The model under review builds one solid part; all positions refer to its coordinate system, in mm. A direction names the side the tool comes from. Give positions to 0.01 mm unless a question says otherwise; leave off trailing zeros. Order: outer loops, then holes, each group sorted by start corner. A loop starts at its lowest first (then second) coordinate and runs counter-clockwise, first axis right, second up. Notation, with made-up numbers: (19.25, -20) - (32.25, -20) arc R21 cw to (32.25, 14) - close; hole circle Ø5 at (-34.5, 64.5). An arc over 180 degrees is marked (long way). Put each result on its own line as item: value.
```python
from build123d import *

# Parameters (mm, degrees)
M4_TAPPED_HOLE1_D     = 3.3
M4_TAPPED_HOLE1_DEPTH = 6
M4_TAPPED_HOLE1_TIP   = 0.991420021
SKETCH6_W             = 40
SKETCH6_H             = 40
BOSS_EXTRUDE1_DEPTH   = 28.5
CUT_EXTRUDE1_REACH    = 124.315
CIRPATTERN1_COUNT     = 4
CHAMFER1_SIZE         = 0.4
BOSS_EXTRUDE2_DEPTH   = 1.5


with BuildPart() as part:
    # Sketch1 → Revolve1 (revolve)
    with BuildSketch(Plane.XY, mode=Mode.PRIVATE) as revolve1_sk:
        Polygon((0, 0), (0, 20), (64.5, 20), (64.5, 13), (66.5, 13), (66.5, 6), (67.5, 6), (67.5, 5), (90.5, 5), (90.5, 0), align=None)
    revolve(revolve1_sk.sketch.rotate(Axis((0, 0, 0), (1, 0, 0)), 90), axis=Axis((0, 0, 0), (1, 0, 0)))

    # M4 Tapped Hole1
    with Locations(Plane(origin=(64.5, 0, 0), x_dir=(0, 0, -1), z_dir=(1, 0, 0))):
        with Locations((12.02081528, -12.02081528), (12.02081528, 12.02081528), (-12.02081528, -12.02081528), (-12.02081528, 12.02081528)):
            Hole(M4_TAPPED_HOLE1_D / 2, depth=M4_TAPPED_HOLE1_DEPTH)
            with Locations((0, 0, -(M4_TAPPED_HOLE1_DEPTH + M4_TAPPED_HOLE1_TIP / 2))):  # 118° drill point
                Cone(0, M4_TAPPED_HOLE1_D / 2, M4_TAPPED_HOLE1_TIP, mode=Mode.SUBTRACT)

    # Sketch6 → Boss-Extrude1 (add)
    with BuildSketch(Plane.ZY):
        Rectangle(SKETCH6_W, SKETCH6_H)
    extrude(amount=BOSS_EXTRUDE1_DEPTH)

    # Sketch7 → Cut-Extrude1 (cut, up to next)
    with BuildSketch(Plane.ZY.offset(28.5), mode=Mode.PRIVATE) as cut_extrude1_sk1:
        with BuildLine():
            Line((-20, 20), (-20, 18.138357147))
            ThreePointArc((-20, 18.138357147), (-19.091883092, 19.091883092), (-18.138357147, 20))
            Line((-18.138357147, 20), (-20, 20))
        make_face()
    cut_extrude1_tool1 = extrude(cut_extrude1_sk1.sketch, amount=-CUT_EXTRUDE1_REACH, mode=Mode.PRIVATE) & part.part
    cut_extrude1 = cut_extrude1_tool1.solids().sort_by_distance((-28.5, 19.389578, -19.389578))[0]
    add(cut_extrude1, mode=Mode.SUBTRACT)

    # CirPattern1: Cut-Extrude1 ×4 about axis
    cirpattern1_axis = Axis((0, 0, 0), (-1, 0, 0))
    for i in range(1, CIRPATTERN1_COUNT):
        add(cut_extrude1.rotate(cirpattern1_axis, i * 360 / CIRPATTERN1_COUNT), mode=Mode.SUBTRACT)

    # Chamfer1
    chamfer1_edges = [part.edges().sort_by_distance(p)[0] for p in [
        (90.5, 0, -5),
    ]]
    chamfer(chamfer1_edges, length=CHAMFER1_SIZE)

    # Sketch8 → Boss-Extrude2 (add, symmetric)
    with BuildSketch(Plane(origin=(0, 5, 0), x_dir=(1, 0, 0), z_dir=(0, 1, 0))):
        with BuildLine():
            Line((71.2, 1.5), (86.8, 1.5))
            ThreePointArc((86.8, 1.5), (87.648528137, 1.148528137), (88, 0.3))
            Line((88, 0.3), (88, -0.3))
            ThreePointArc((88, -0.3), (87.648528137, -1.148528137), (86.8, -1.5))
            Line((86.8, -1.5), (71.2, -1.5))
            ThreePointArc((71.2, -1.5), (70.351471863, -1.148528137), (70, -0.3))
            Line((70, -0.3), (70, 0.3))
            ThreePointArc((70, 0.3), (70.351471863, 1.148528137), (71.2, 1.5))
        make_face()
    extrude(amount=BOSS_EXTRUDE2_DEPTH, both=True)


solid = part.part
```
(1) Clearance check with flat-ended pins moving along their axes: pin 1 Ø0.5 at (x, y) = (82, 6) entering from +Z; pin 2 Ø2 at (x, y) = (7.5, -12.5) entering from -Z; pin 3 Ø6 at (y, z) = (-4, -12.5) entering from +X. State where each tip first meets the part, or that it passes through.
The answers:
pin 1: z = 1.5
pin 2: z = -16.36
pin 3: x = 66.5
(2) Take a section at A-A, the plane y = -15.5. Write out the cut boundary in (x, z), then the cut area to 3 significant figures.
The answers:
outline: (-28.5, -20) - (0, -20) - (0, -12.64) - (64.5, -12.64) - (64.5, 12.64) - (0, 12.64) - (0, 20) - (-28.5, 20) - close
area: 2,770 mm^2
(3) The part is to be moulded in two halves that separate along Z. For faces 6 (the cylindrical face through (65.514, 7.91, -10.316)), 7 (the flat face through (0, 15, 15)), 8 (the cylindrical face through (61.46, 13.41, -11.13)), say which applies: pulls with the +Z half, pulls with the -Z half, needs draft (parallel to the pull), parting line crosses it, or undercut.
The answers:
face 6: parting line crosses it
face 7: needs draft
face 8: undercut
(4) Take a section at B-B, the plane z = -7.5. Write out the cut boundary in (x, y).
The answers:
outline: (-28.5, -20) - (0, -20) - (0, -18.54) - (64.5, -18.54) - (64.5, -10.62) - (66.5, -10.62) - (66.5, 10.62) - (64.5, 10.62) - (64.5, 18.54) - (0, 18.54) - (0, 20) - (-28.5, 20) - close
(5) Take a section at D-D, the plane y = 15. Write out the cut boundary in (x, z).
The answers:
outline: (-28.5, -20) - (0, -20) - (0, -13.23) - (64.5, -13.23) - (64.5, 13.23) - (0, 13.23) - (0, 20) - (-28.5, 20) - close
(6) For faces 1 (the flat face through (-14, -20, 0)), 2 (the flat face through (79, 6.5, 0)), 3 (the cylindrical face through (61.458, -12.653, -10.497)), 4 (the flat face through (-14, 0, 20)), 5 (the flat face through (0, -15, -16)), list the 3-axis set-ups (+Z, -Z, +X, -X, +Y, -Y) from which the entire face can be reached by the end or side of a thin tool; tool diameter is ignored.
The answers:
face 1: +Z, -Z, +X, -X, -Y
face 2: +Z, -Z, +X, +Y
face 3: +X
face 4: +Z, +X, -X, +Y, -Y
face 5: -Z, +X, -Y
(7) Take a section at C-C, the plane x = 47. Write out the cut boundary in (y, z), then the cut area to 3 significant figures.
The answers:
outline: circle Ø40 at (0, 0)
area: 1,260 mm^2
(8) Wall thickness on L1, parallel to X at y = -9, z = 16.5; L2, parallel to X at y = 12.5, z = -16; L3, parallel to Z at x = 15, y = -2.5: over which ranges is each line inside the solid? List them lowest first.
The answers:
L1: -28.5 to 64.5
L2: -28.5 to 0
L3: -19.84 to 19.84
